```python
from build123d import *

# Parameters (mm, degrees)
BOSS_EXTRUDE1_DEPTH                            = 10
SKETCH2_W                                      = 5.125
SKETCH2_H                                      = 10
CUT_EXTRUDE1_DEPTH                             = 4
CSK_FOR_M2_FLAT_HEAD_MACHINE_SCREW1_AT_2_COUNT = 2
CSK_FOR_M2_FLAT_HEAD_MACHINE_SCREW1_AT_2_PITCH = 14


with BuildPart() as part:
    # Sketch1 → Boss-Extrude1 (new body, symmetric)
    with BuildSketch(Plane(origin=(0, 0, 0), x_dir=(0, 0, -1), z_dir=(1, 0, 0))):
        Polygon((0, 0), (10, 0), (10, -3), (-3, -3), (-3, 5), (0, 5), align=None)
    extrude(amount=BOSS_EXTRUDE1_DEPTH, both=True)

    # Sketch2 → Cut-Extrude1 (cut, through all)
    with BuildSketch(Plane(origin=(0, 0, 0), x_dir=(1, 0, 0), z_dir=(0, 1, 0))):
        with Locations((-7.4375, 5)):
            Rectangle(SKETCH2_W, SKETCH2_H)
        with Locations((7.4375, 5)):
            Rectangle(SKETCH2_W, SKETCH2_H)
    extrude(amount=-CUT_EXTRUDE1_DEPTH, mode=Mode.SUBTRACT)

    # Sketch4 → CSK for M2 Flat Head Machine Screw1 (revolve, cut)
    with BuildSketch(Plane(origin=(7, 2.5, 3), x_dir=(0, -1, 0), z_dir=(1, 0, 0))):
        Polygon((0, 0), (0, 20.721032743), (1.2, 20), (1.2, 1.15), (2.2, 0.15), (2.2, 0), align=None)
    csk_for_m2_flat_head_machine_screw1 = revolve(axis=Axis((7, 2.5, 9.35), (0, 0, -1)), mode=Mode.SUBTRACT)

    # CSK for M2 Flat Head Machine Screw1 at 2: CSK for M2 Flat Head Machine Screw1 ×2
    with Locations(*[(-i * CSK_FOR_M2_FLAT_HEAD_MACHINE_SCREW1_AT_2_PITCH, 0, 0) for i in range(1, CSK_FOR_M2_FLAT_HEAD_MACHINE_SCREW1_AT_2_COUNT)]):
        add(csk_for_m2_flat_head_machine_screw1, mode=Mode.SUBTRACT)


solid = part.part
```
The listing builds one solid part. Answer for the finished solid, in the listing's coordinates (mm). A direction names the side the tool comes from. Coordinates: 2 decimals unless noted, no trailing zeros. Loops run counter-clockwise (first coordinate to the right, second up) from the corner with the lowest first, then second, coordinate; pieces in that order, holes last. Notation, with made-up numbers: (78.5, 25.5) -> (126.5, 25.5) arc R30 cw to (126.5, 61.5) -> close; hole circle Ø6 at (43, -23). An arc over 180 degrees is marked (long way). Return JSON: item names as keys, results as strings. Group by question number.
(1) Given pin 1 Ø2.5 at (y, z) = (-1.5, -4) entering from +X (3 decimals); pin 2 Ø3 at (x, z) = (-5.5, -4) entering from +Y; pin 3 Ø2.5 at (y, z) = (-1.5, -7.5) entering from -X (3 decimals); pin 4 Ø2 at (x, y) = (7, 2.5) entering from -Z, each flat-ended and moving along its own axis, determine where each tip first touches the part or whether it passes through.
(2) Which of the six approach directions +Z, -Z, +X, -X, +Y, -Y give full straight-line access (tool end or side, diameter ignored) to faces 1 (the flat face through (-10, 1, 1)), 2 (the flat face through (-4.875, -1, -5))?
(3) A cutting plane is placed at A-A on y = 2.5. Write down the section's boundary in (x, z).
(4) A cutting plane is placed at B-B on x = -7. Write down the section's boundary in (y, z).
(5) A cutting plane is placed at D-D on z = 0.5. Write down the section's boundary in (x, y), and give its area (3 significant figures).
(6) Find the intervals of material crossed by probe 1 along X at (y, z) = (2.5, 2.9); probe 2 along Y at (x, z) = (-7, 2.9); probe 3 along Y at (x, z) = (-4.75, -0.5), in increasing order. Write a range as from..to.
(7) A cutting plane is placed at C-C on y = -1.75. Write down the section's boundary in (x, z) (3 decimals), and give its area (4 significant figures).
(8) Determine the mould class of faces 3 (the cylindrical face through (-8.19, 2.66, 0.94)), 4 (the flat face through (4.875, -1, -5)), 5 (the flat face through (0, 0, -5)) for opening direction Y: released by +Y, released by -Y, zero draft, split by the parting line, or undercut.
The answers:
{
 "1": {"pin 1": "stops at x = 4.875", "pin 2": "stops at y = 0", "pin 3": "stops at x = -4.875", "pin 4": "passes through"},
 "2": {"face 1": "+Z, -Z, -X, +Y, -Y", "face 2": "-Z, -X, +Y, -Y"},
 "3": {"outline": "(-10, 0) -> (-8.2, 0) -> (-8.2, 1.85) -> (-9.2, 2.85) -> (-9.2, 3) -> (-10, 3) -> close; (-5.8, 0) -> (5.8, 0) -> (5.8, 1.85) -> (4.8, 2.85) -> (4.8, 3) -> (-4.8, 3) -> (-4.8, 2.85) -> (-5.8, 1.85) -> close; (8.2, 0) -> (10, 0) -> (10, 3) -> (9.2, 3) -> (9.2, 2.85) -> (8.2, 1.85) -> close"},
 "4": {"outline": "(-3, 0) -> (1.3, 0) -> (1.3, 1.85) -> (0.3, 2.85) -> (0.3, 3) -> (-3, 3) -> close; (3.7, 0) -> (5, 0) -> (5, 3) -> (4.7, 3) -> (4.7, 2.85) -> (3.7, 1.85) -> close"},
 "5": {"outline": "(-10, -3) -> (10, -3) -> (10, 5) -> (-10, 5) -> close; hole circle Ø2.4 at (-7, 2.5); hole circle Ø2.4 at (7, 2.5)", "area": "151 mm^2"},
 "6": {"probe 1": "x = -10..-9.2, -4.8..4.8, 9.2..10", "probe 2": "y = -3..0.3, 4.7..5", "probe 3": "y = -3..0"},
 "7": {"outline": "(-10, 0) -> (-4.875, 0) -> (-4.875, -10) -> (4.875, -10) -> (4.875, 0) -> (10, 0) -> (10, 3) -> (-10, 3) -> close", "area": "157.5 mm^2"},
 "8": {"face 3": "undercut", "face 4": "zero draft", "face 5": "released by +Y"}
}
